from build123d import *

# Parameters (mm, degrees)
BOSS_EXTRUDE1_DEPTH     = 40
SKETCH2_R               = 43
SKETCH2_R_2             = 35
CUT_EXTRUDE1_DEPTH      = 5
SKETCH2_5_R             = 35
CUT_EXTRUDE2_DEPTH      = 1
CUT_EXTRUDE2_DEPTH_BACK = 41
SKETCH4_R               = 35
BOSS_EXTRUDE3_DEPTH     = 20
SKETCH4_4_R             = 25
BOSS_EXTRUDE4_DEPTH     = 90


with BuildPart() as part:
    # Sketch1 → Boss-Extrude1 (new body)
    with BuildSketch(Plane.XY):
        with BuildLine():
            ThreePointArc((56.338184709, -20.639984102), (0, 60), (-56.338184709, -20.639984102))
            ThreePointArc((-56.338184709, -20.639984102), (-50, -100), (-56.338184709, -179.360015898))
            ThreePointArc((-56.338184709, -179.360015898), (0, -260), (56.338184709, -179.360015898))
            ThreePointArc((56.338184709, -179.360015898), (50, -100), (56.338184709, -20.639984102))
        make_face()
    extrude(amount=-BOSS_EXTRUDE1_DEPTH)

    # Sketch2 → Cut-Extrude1 (cut)
    with BuildSketch(Plane.XY):
        with Locations((0, -100)):
            Circle(SKETCH2_R)
        with Locations((0, -100)):
            Circle(SKETCH2_R_2, mode=Mode.SUBTRACT)
        with BuildLine():
            ThreePointArc((7.008521599, -42.425), (0, 43), (-7.008521599, -42.425))
            ThreePointArc((-7.008521599, -42.425), (-26.989032945, -48.661981917), (-43.454545455, -61.585126847))
            ThreePointArc((-43.454545455, -61.585126847), (-45.552404101, -40.028148339), (-48.567238975, -18.580185639))
            ThreePointArc((-48.567238975, -18.580185639), (0, 52), (48.567238975, -18.580185639))
            ThreePointArc((48.567238975, -18.580185639), (45.552404101, -40.028148339), (43.454545455, -61.585126847))
            ThreePointArc((43.454545455, -61.585126847), (26.989032945, -48.661981917), (7.008521599, -42.425))
        make_face()
        with BuildLine():
            ThreePointArc((7.008521599, -157.575), (26.989032945, -151.338018083), (43.454545455, -138.414873153))
            ThreePointArc((43.454545455, -138.414873153), (45.552404101, -159.971851661), (48.567238975, -181.419814361))
            ThreePointArc((48.567238975, -181.419814361), (0, -252), (-48.567238975, -181.419814361))
            ThreePointArc((-48.567238975, -181.419814361), (-45.552404101, -159.971851661), (-43.454545455, -138.414873153))
            ThreePointArc((-43.454545455, -138.414873153), (-26.989032945, -151.338018083), (-7.008521599, -157.575))
            ThreePointArc((-7.008521599, -157.575), (0, -243), (7.008521599, -157.575))
        make_face()
    extrude(amount=-CUT_EXTRUDE1_DEPTH, mode=Mode.SUBTRACT)

    # Sketch2<5> → Cut-Extrude2 (cut, two sides)
    with BuildSketch(Plane.XY) as cut_extrude2_sk:
        Circle(SKETCH2_5_R)
        with Locations((0, -200)):
            Circle(SKETCH2_5_R)
    extrude(amount=CUT_EXTRUDE2_DEPTH, mode=Mode.SUBTRACT)
    extrude(cut_extrude2_sk.sketch, amount=-CUT_EXTRUDE2_DEPTH_BACK, mode=Mode.SUBTRACT)

    # Sketch4 → Boss-Extrude3 (add)
    with BuildSketch(Plane(origin=(0, 0, -40), x_dir=(-1, 0, 0), z_dir=(0, 0, -1))):
        with Locations((0, -100)):
            Circle(SKETCH4_R)
    extrude(amount=BOSS_EXTRUDE3_DEPTH)

    # Sketch4<4> → Boss-Extrude4 (add)
    with BuildSketch(Plane(origin=(0, 0, -40), x_dir=(-1, 0, 0), z_dir=(0, 0, -1))):
        with Locations((0, -100)):
            Circle(SKETCH4_4_R)
    extrude(amount=BOSS_EXTRUDE4_DEPTH)


solid = part.part
Read the model definition and answer for the solid it produces. Units are mm, in the model's axes. A direction names the side the tool comes from. Give positions to 0.01 mm unless a question says otherwise; leave off trailing zeros. Write each loop counter-clockwise with the first axis right and the second up, starting at its lowest first coordinate (ties: lowest second). Pieces come first, ordered by that corner, then holes. Notation, with made-up numbers: (13, -25) -> (21, -25) arc R4 ccw to (21, -20) -> close; hole circle Ø5 at (55.5, -8). An arc over 180 degrees is marked (long way). Answer as a JSON object with one key per item and string values. Group by question number.
1) Find section C-C (x = 0). Count the separate pieces of the cut face and the enclosed holes in it, and give its area (3 significant figures).
2) The mould has two halves that part along X. Classify faces 4 (the flat face through (0, -100, 0)), 5 (the flat face through (12, -42, -5)), 6 (the cylindrical face through (50, -101, -20)), 7 (the cylindrical face through (4.56, -65.3, -49.86)): +X half, -X half, draft (parallel to the pull), parting line (faces both ways), or undercut.
3) Find section D-D (z = -87). Write down the section's boundary in (x, y).
4) Each of these flat-tipped pins is pushed along its axis until it touches: P1, Ø8, axis at y = -85, z = -60.5, coming from the -X side; P2, Ø6, axis at x = -10, z = -34, coming from the +Y side; P3, Ø4, axis at y = -93, z = -35.5, coming from the +X side. Where does it stop, or does it pass through?
5) Consider L1, parallel to Y at x = 0, z = -15; L2, parallel to Y at x = 30.5, z = -19; L3, parallel to Z at x = -52, y = -158.5. Determine where each line is inside the solid, lowest interval first. Write a range as from..to.
6) Find section A-A (y = -200). Write down the section's boundary in (x, z), and give its area (3 significant figures).
7) Find section B-B (y = -100). Write down the section's boundary in (x, z), and give its area (3 significant figures).
8) A tool of negligible diameter and unlimited length cuts with its end or side. For faces 1 (the cylindrical face through (1.61, 59.98, -19.72)), 2 (the cylindrical face through (-9.322, -141.977, -2.465)), 3 (the cylindrical face through (5.42, -124.406, -94.51)), from which of +Z, -Z, +X, -X, +Y, -Y can it reach the whole face along a straight path? Write none if from no direction.
Values follow:
{
 "1": {"separate pieces": "3", "enclosed holes": "0", "area": "11,900 mm2"},
 "2": {"face 4": "draft", "face 5": "undercut", "face 6": "+X half", "face 7": "parting line"},
 "3": {"outline": "circle Ø50 at (0, -100)"},
 "4": {"P1": "stops at x = -33.22", "P2": "stops at y = 59.59", "P3": "stops at x = 50.08"},
 "5": {"L1": "y = -260..-235, -165..-35, 35..60", "L2": "y = -251.67..-217.17, -182.83..-17.17, 17.17..51.67", "L3": "z = -40..0"},
 "6": {"outline": "(-60, -40) -> (-35, -40) -> (-35, 0) -> (-43, 0) -> (-43, -5) -> (-52, -5) -> (-52, 0) -> (-60, 0) -> close; (35, -40) -> (60, -40) -> (60, 0) -> (52, 0) -> (52, -5) -> (43, -5) -> (43, 0) -> (35, 0) -> close", "area": "1,910 mm2"},
 "7": {"outline": "(-50, -40) -> (-35, -40) -> (-35, -60) -> (-25, -60) -> (-25, -130) -> (25, -130) -> (25, -60) -> (35, -60) -> (35, -40) -> (50, -40) -> (50, 0) -> (43, 0) -> (43, -5) -> (35, -5) -> (35, 0) -> (-35, 0) -> (-35, -5) -> (-43, -5) -> (-43, 0) -> (-50, 0) -> close", "area": "8,820 mm2"},
 "8": {"face 1": "+Z, -Z", "face 2": "+Z", "face 3": "-Z"}
}
